from build123d import *

# Parameters (mm, degrees)
SKETCH1_R           = 1.15
BOSS_EXTRUDE1_DEPTH = 3


with BuildPart() as part:
    # Sketch1 → Boss-Extrude1 (new body)
    with BuildSketch(Plane.XY):
        with BuildLine():
            Line((-2.923110194, -0.674853163), (-5.903711664, 12.235550195))
            ThreePointArc((-5.903711664, 12.235550195), (-5.961317037, 12.570793717), (-5.98060147, 12.910403358))
            Line((-5.98060147, 12.910403358), (-5.98060147, 27.910403358))
            ThreePointArc((-5.98060147, 27.910403358), (-2.98060147, 30.910403358), (0.01939853, 27.910403358))
            Line((0.01939853, 27.910403358), (0.01939853, 13.252210183))
            Line((0.01939853, 13.252210183), (2.923110194, 0.674853163))
            ThreePointArc((2.923110194, 0.674853163), (0.674853163, -2.923110194), (-2.923110194, -0.674853163))
        make_face()
        Circle(SKETCH1_R, mode=Mode.SUBTRACT)
        with Locations((-1.82210354, 7.892397525)):
            Circle(SKETCH1_R, mode=Mode.SUBTRACT)
    extrude(amount=BOSS_EXTRUDE1_DEPTH)


solid = part.part
Geometry check sheet. Reference: the model listing, model coordinates, mm. A direction names the side the tool comes from. Round coordinates to 2 decimals unless told otherwise and drop trailing zeros. Loops run counter-clockwise (first coordinate to the right, second up) from the corner with the lowest first, then second, coordinate; pieces in that order, holes last. Notation, with made-up numbers: (-3.5, 24.25) -> (21.5, 24.25) arc R25 cw to (21.5, 36.25) -> close; hole circle Ø3 at (-14.75, -1.75). An arc over 180 degrees is marked (long way). Answer as a JSON object with one key per item and string values. Group by question number.
Item 1: Thickness scan on line 1 along X through (y, z) = (18.5, 2.05); line 2 along X through (y, z) = (0.5, 2.5); line 3 along X through (y, z) = (8.5, 1.5). Record the ranges inside material, lowest first.
Item 2: Cross-section at C-C, the plane z = 2.25. Record the cut outline in (x, y).
Item 3: Cross-section at D-D, the plane y = 26.5. Record the cut outline in (x, z), plus the area to 3 significant figures.
Item 4: Depth check by flat-ended pin: pin 1 Ø1.5 at (y, z) = (20.5, 1) entering from +X; pin 2 Ø1 at (x, z) = (-1, 1.5) entering from -Y. Enter the tip coordinate at first touch or a pass-through.
Item 5: Cross-section at A-A, the plane y = 0. Record the cut outline in (x, z).
Item 6: Release check for a two-part mould opening along X. For faces 3 (the face through (-0.91, -0.7, 1.48)), 4 (the face through (0.739, -2.908, 1.479)), 5 (the face through (-2, 14, 0)) record: pulls with the +X half, pulls with the -X half, needs draft (parallel to the pull), parting line crosses it, or undercut.
Item 7: Set-up check for faces 1 (the face through (-5.981, 20, 1)), 2 (the face through (0.019, 21, 1)): record each of +Z, -Z, +X, -X, +Y, -Y from which the full face is reachable in a straight line by a thin tool's end or side.
Item 8: Cross-section at B-B, the plane x = -2.25. Record the cut outline in (y, z), plus the area to 3 significant figures.
Determined:
{
 "1": {"line 1": "x = -5.98 to 0.02", "line 2": "x = -3.19 to -1.04, 1.04 to 2.96", "line 3": "x = -5.04 to -2.8, -0.85 to 1.12"},
 "2": {"outline": "(-5.98, 12.91) arc R3 ccw to (-5.9, 12.24) -> (-2.92, -0.67) arc R3 ccw to (2.92, 0.67) -> (0.02, 13.25) -> (0.02, 27.91) arc R3 ccw to (-5.98, 27.91) -> close; hole circle Ø2.3 at (-1.82, 7.89); hole circle Ø2.3 at (0, 0)"},
 "3": {"outline": "(-5.98, 0) -> (0.02, 0) -> (0.02, 3) -> (-5.98, 3) -> close", "area": "18.0 mm²"},
 "4": {"pin 1": "stops at x = 0.02", "pin 2": "stops at y = -2.96"},
 "5": {"outline": "(-3.08, 0) -> (-1.15, 0) -> (-1.15, 3) -> (-3.08, 3) -> close; (1.15, 0) -> (3, 0) -> (3, 3) -> (1.15, 3) -> close"},
 "6": {"face 3": "undercut", "face 4": "parting line crosses it", "face 5": "needs draft"},
 "7": {"face 1": "+Z, -Z, -X, +Y, -Y", "face 2": "+Z, -Z, +X, +Y"},
 "8": {"outline": "(-1.98, 0) -> (6.82, 0) -> (6.82, 3) -> (-1.98, 3) -> close; (8.96, 0) -> (30.82, 0) -> (30.82, 3) -> (8.96, 3) -> close", "area": "92.0 mm²"}
}
